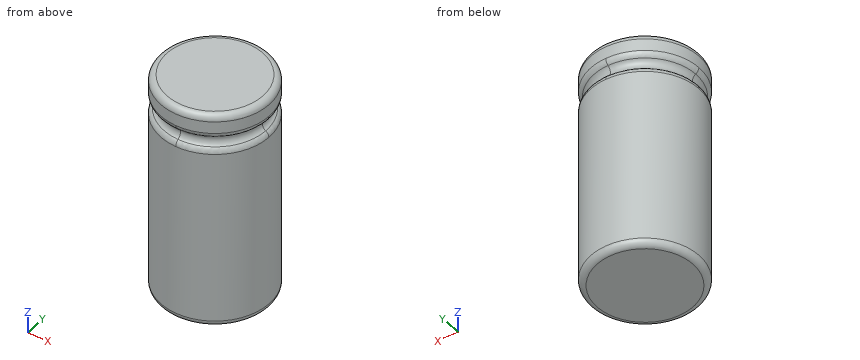
from build123d import *

# Parameters (mm, degrees)
SKETCH1_R           = 17.5
BOSS_EXTRUDE1_DEPTH = 71
FILLET1_R           = 2
SKETCH2_R           = 2.061113782
FILLET2_R           = 2


with BuildPart() as part:
    # Sketch1 → Boss-Extrude1 (new body)
    with BuildSketch(Plane.XY):
        Circle(SKETCH1_R)
    extrude(amount=BOSS_EXTRUDE1_DEPTH)

    # Fillet1
    fillet1_edges = [part.edges().sort_by_distance(p)[0] for p in [
        (-17.5, 0, 0),
        (-17.5, 0, 71),
    ]]
    fillet(fillet1_edges, radius=FILLET1_R)

    # Cut-Sweep1: sweep along a curve in space
    with BuildLine() as cut_sweep1_path:
        ThreePointArc((17.5, 0, 69), (12.374368671, 12.374368671, 69), (0, 17.5, 69))
        ThreePointArc((0, 17.5, 69), (-12.374368671, 12.374368671, 69), (-17.5, 0, 69))
        ThreePointArc((-17.5, 0, 69), (-12.374368671, -12.374368671, 69), (0, -17.5, 69))
        ThreePointArc((0, -17.5, 69), (12.374368671, -12.374368671, 69), (17.5, 0, 69))
    # Sketch2 → Cut-Sweep1 (sweep, cut)
    with BuildSketch(Plane(origin=(0, 0, 0), x_dir=(1, 0, 0), z_dir=(0, 1, 0))):
        with Locations((17.5, -61.590274305)):
            Circle(SKETCH2_R)
    sweep(path=cut_sweep1_path.line, mode=Mode.SUBTRACT)

    # Fillet2
    fillet2_edges = [part.edges().sort_by_distance(p)[0] for p in [
        (-12.374368671, -12.374368671, 63.651388087),
        (12.374368671, -12.374368671, 59.529160523),
    ]]
    fillet(fillet2_edges, radius=FILLET2_R)


solid = part.part
Model file for the job. Use its own axes, mm. Give positions to 0.01 mm unless a question says otherwise; leave off trailing zeros. Loops run counter-clockwise (first coordinate to the right, second up) from the corner with the lowest first, then second, coordinate; pieces in that order, holes last.
1) Wall check: line 1 (Z direction, x = -9.5, y = -12.5); line 2 (Z direction, x = 4.5, y = -16); line 3 (Y direction, x = 5, z = 36.5). Give the ranges that are in metal, low to high.
2) Flat gauge pins, fed straight in: pin 1 Ø12 at (x, z) = (11.5, 8) entering from +Y; pin 2 Ø3 at (x, z) = (-5, 41) entering from -Y; pin 3 Ø5 at (y, z) = (6, 8) entering from -X. Where does each tip first touch, or does it go through?
3) Saw through at A-A (z = 30.5). Write the cut outline in (x, y), plus the area to 3 significant figures.
Answer block:
1. line 1: z = 0.01 to 60.59, 62.59 to 70.99
1. line 2: z = 0.34 to 59.71, 63.47 to 70.66
1. line 3: y = -16.77 to 16.77
2. pin 1: stops at y = 16.61
2. pin 2: stops at y = -17.15
2. pin 3: stops at x = -17.15
3. outline: circle Ø35 at (0, 0)
3. area: 962 mm2
